Source: CAD feature listing. Evaluate the final solid. Frame: model axes, mm. A direction names the side the tool comes from. Give positions to 0.01 mm unless a question says otherwise; leave off trailing zeros. Order: outer loops, then holes, each group sorted by start corner. A loop starts at its lowest first (then second) coordinate and runs counter-clockwise, first axis right, second up. Notation, with made-up numbers: M 36,80 L 60,80 A13 ccw 60,89 Z; hole C -19.5,75.25 d1. An arc over 180 degrees is marked long. Use CSV: the item, a comma, the result in double quotes. Start each with the question number.
Item 1: Section query C-C on y = 10. Return loops of the section in (x, z).
Item 2: Section query A-A on x = 21.5. Return loops of the section in (y, z).
Item 3: Ray query, probe 1 along Y at (x, z) = (0, -11.75); probe 2 along Z at (x, y) = (0.5, 17.5); probe 3 along Y at (x, z) = (-18.5, 2.5). Return the intervals inside material, ascending. Write a range as from..to.
Item 4: Section query B-B on y = 2.75. Return loops of the section in (x, z).
Item 5: Section query D-D on x = -21. Return loops of the section in (y, z).
Item 6: First-contact query: pin 1 (4 mm diameter, centred on y = 10, z = 0, fed in from +X); pin 2 (1 mm diameter, centred on y = 12.5, z = -4.5, fed in from +X); pin 3 (5 mm diameter, centred on x = -14, z = -7.5, fed in from -Y). Flat tips, straight axial feed; report the tip coordinate or a pass-through.
Item 7: Access query for faces 5 (the face through (-11.882, 4.535, 22.845)), 6 (the face through (1.4, 16.93, -10.66)), 7 (the face through (18, 7, 5)), 8 (the face through (11, 2, 0)), 9 (the face through (-10.459, 8.536, 0.325)). Directions: +Z, -Z, +X, -X, +Y, -Y. A direction counts if a zero-diameter tool reaches every point of the face in a straight line with its end or side. Return the directions, or none.
Item 8: Pull-direction query (X, two-part tool) for faces 1 (the face through (-2, 12, -3)), 2 (the face through (-11, 22, 0)), 3 (the face through (0.325, 8.536, -10.675)), 4 (the face through (1.4, 1.01, -10.66)); classes: +X half, -X half, draft (parallel to the pull), parting line (faces both ways), or undercut.
from build123d import *

# Parameters (mm, degrees)
SKETCH3_R          = 0.5
SKETCH3_R_2        = 1.5
CUT_EXTRUDE1_DEPTH = 43.545563811
CIRPATTERN1_COUNT  = 2
CIRPATTERN1_ANGLE  = 90
SKETCH4_R          = 1.5
CUT_EXTRUDE2_DEPTH = 13


with BuildPart() as part:
    # Sketch2 → Revolve1 (revolve)
    with BuildSketch(Plane.XY, mode=Mode.PRIVATE) as revolve1_sk:
        Polygon((3.25, 0), (10.75, 0), (10.75, 2), (25.75, 2), (25.75, 7), (18.25, 7), (18.25, 17), (25.75, 17), (25.75, 22), (10.75, 22), (10.75, 12), (3.25, 12), align=None)
    revolve(revolve1_sk.sketch.rotate(Axis((0, 87.545500491, 0), (0, -1, 0)), 180), axis=Axis((0, 87.545500491, 0), (0, -1, 0)))

    # Sketch3 → Cut-Extrude1 (cut, symmetric)
    with BuildSketch(Plane(origin=(0, 0, 0), x_dir=(0, 0, -1), z_dir=(1, 0, 0))):
        with Locations((0, 13)):
            Circle(SKETCH3_R)
        with Locations((0, 16)):
            Circle(SKETCH3_R)
        with Locations((0, 10)):
            Circle(SKETCH3_R_2)
    cut_extrude1 = extrude(amount=CUT_EXTRUDE1_DEPTH, both=True, mode=Mode.SUBTRACT)

    # CirPattern1: Cut-Extrude1 ×2 about axis
    cirpattern1_axis = Axis((0, 22, 0), (0, 1, 0))
    for i in range(1, CIRPATTERN1_COUNT):
        add(cut_extrude1.rotate(cirpattern1_axis, i * CIRPATTERN1_ANGLE / (CIRPATTERN1_COUNT - 1)), mode=Mode.SUBTRACT)

    # Sketch4 → Cut-Extrude2 (cut)
    with BuildSketch(Plane(origin=(0, 22, 0), x_dir=(1, 0, 0), z_dir=(0, 1, 0))):
        with Locations(Location((15.0260191, 15.0260191, 0), (0, 0, 180))):
            Circle(SKETCH4_R)
        with Locations(Location((-15.0260191, -15.0260191, 0), (0, 0, 180))):
            Circle(SKETCH4_R)
    extrude(amount=-CUT_EXTRUDE2_DEPTH, mode=Mode.SUBTRACT)


solid = part.part
Verdict:
1,outline,"M -18.19,-1.5 A18.25 ccw -1.5,-18.19 L -1.5,-2.88 A3.25 cw -2.88,-1.5 Z; M -18.19,1.5 L -2.88,1.5 A3.25 cw -1.5,2.88 L -1.5,18.19 A18.25 ccw Z; M 1.5,-18.19 A18.25 ccw 18.19,-1.5 L 2.88,-1.5 A3.25 cw 1.5,-2.88 Z; M 1.5,2.88 A3.25 cw 2.88,1.5 L 18.19,1.5 A18.25 ccw 1.5,18.19 Z"
2,outline,"M 2,-14.17 L 7,-14.17 L 7,14.17 L 2,14.17 Z; M 17,-14.17 L 22,-14.17 L 22,14.17 L 17,14.17 Z"
3,probe 1,"2..8.5, 11.5..12.5, 13.5..15.5, 16.5..22"
3,probe 2,"-25.75..-10.74, 10.74..25.75"
3,probe 3,"2..7, 17..22"
4,outline,"C 0,0 d51.5; hole C 0,0 d6.5"
5,outline,"M 2,-14.9 L 7,-14.9 L 7,14.9 L 2,14.9 Z; M 17,-14.9 L 22,-14.9 L 22,14.9 L 17,14.9 Z"
6,pin 1,"x = 18.25"
6,pin 2,"x = 17.81"
6,pin 3,"y = 2"
7,face 5,"+Y, -Y"
7,face 6,"+Y"
7,face 7,"none"
7,face 8,"-Y"
7,face 9,"+X, -X"
8,face 1,"undercut"
8,face 2,"draft"
8,face 3,"undercut"
8,face 4,"parting line"
